For this review, use the dimensioned drawing (mm, ordinates from the lowest corner) and the shaded views. A direction names the side the tool comes from. Round coordinates to 2 decimals unless told otherwise and drop trailing zeros. Loops run counter-clockwise (first coordinate to the right, second up) from the corner with the lowest first, then second, coordinate; pieces in that order, holes last. Notation, with made-up numbers: (19.5, 22) -> (61.5, 22) arc R15 ccw to (61.5, 31) -> close; hole circle Ø1 at (41.5, 2.25). An arc over 180 degrees is marked (long way). Answer as CSV lines item,"result". Start each with the question number.
(1) To check wall thickness, follow line 1 (X direction, y = 4, z = 1); line 2 (X direction, y = 2.75, z = 4.2); line 3 (Z direction, x = 14.5, y = 4.5). State the ranges of each line that lie inside material, in increasing order. Write a range as from..to.
(2) Take a section at C-C, the plane y = 3.9. Write out the cut boundary in (x, z).
(3) Draft analysis for pull direction X (two halves, no side actions). For the marked faces 4, 5, 6 and 7, state which applies: +X half, -X half, draft (parallel to the pull), parting line (faces both ways), or undercut.
(4) For P1, Ø4, axis at x = 13, y = 3, coming from the +Z side; P2, Ø1.5, axis at x = 3, y = 4, coming from the +Z side, all flat-tipped, find the tip position at first contact; note any pin that passes through.
(5) Machinability: for the marked faces 1, 2 and 3, which of the approach directions +Z, -Z, +X, -X, +Y, -Y give a long, thin tool a straight path to every point of the face, cutting with its end or side? Answer none if there is none.
(6) Take a section at A-A, the plane z = 3.4. Write out the cut boundary in (x, y), and give its area (3 significant figures).
(7) Take a section at D-D, the plane z = 1.3. Write out the cut boundary in (x, y).
(8) Take a section at B-B, the plane x = 11.9. Write out the cut boundary in (y, z), and give its area (3 significant figures).
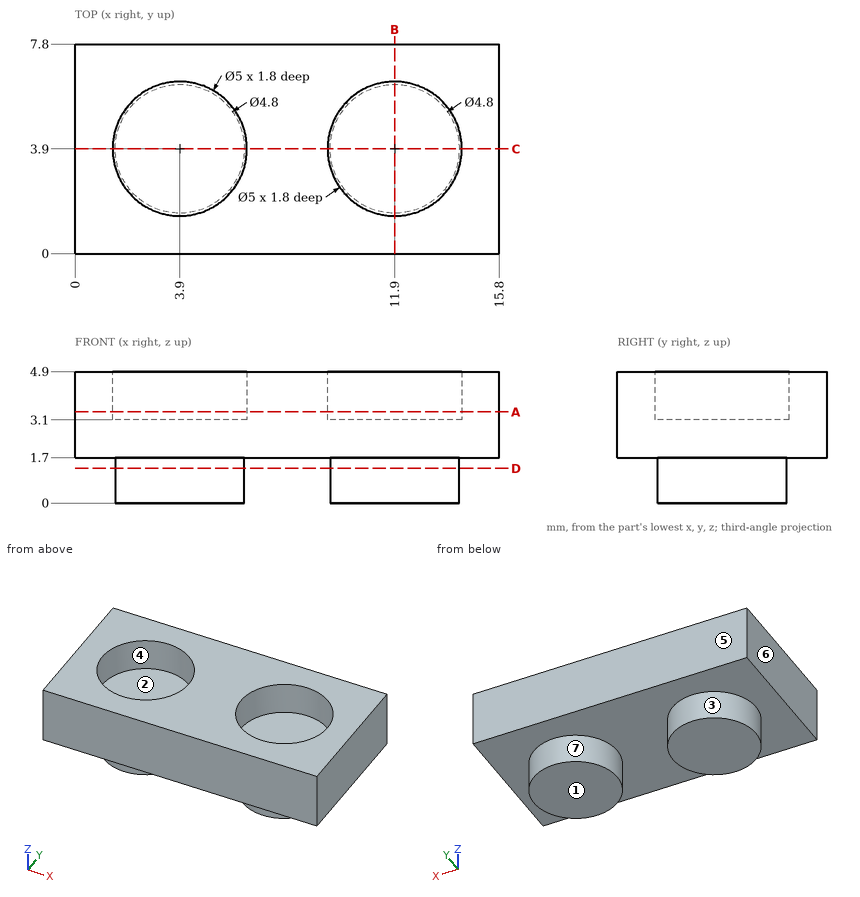
The answers:
1,line 1,"1.5..6.3, 9.5..14.3"
1,line 2,"0..1.68, 6.12..9.68, 14.12..15.8"
1,line 3,"1.7..4.9"
2,outline,"(0, 1.7) -> (1.5, 1.7) -> (1.5, 0) -> (6.3, 0) -> (6.3, 1.7) -> (9.5, 1.7) -> (9.5, 0) -> (14.3, 0) -> (14.3, 1.7) -> (15.8, 1.7) -> (15.8, 4.9) -> (14.4, 4.9) -> (14.4, 3.1) -> (9.4, 3.1) -> (9.4, 4.9) -> (6.4, 4.9) -> (6.4, 3.1) -> (1.4, 3.1) -> (1.4, 4.9) -> (0, 4.9) -> close"
3,face 4,"undercut"
3,face 5,"draft"
3,face 6,"-X half"
3,face 7,"undercut"
4,P1,"z = 4.9"
4,P2,"z = 3.1"
5,face 1,"-Z, +X, -X, +Y, -Y"
5,face 2,"+Z"
5,face 3,"-Z"
6,outline,"(0, 0) -> (15.8, 0) -> (15.8, 7.8) -> (0, 7.8) -> close; hole circle Ø5 at (3.9, 3.9); hole circle Ø5 at (11.9, 3.9)"
6,area,"84.0 mm²"
7,outline,"circle Ø4.8 at (3.9, 3.9); circle Ø4.8 at (11.9, 3.9)"
8,outline,"(0, 1.7) -> (1.5, 1.7) -> (1.5, 0) -> (6.3, 0) -> (6.3, 1.7) -> (7.8, 1.7) -> (7.8, 4.9) -> (6.4, 4.9) -> (6.4, 3.1) -> (1.4, 3.1) -> (1.4, 4.9) -> (0, 4.9) -> close"
8,area,"24.1 mm²"
